Can you work these out from the model? Positions are in its coordinate system, mm. A direction names the side the tool comes from. Round coordinates to 2 decimals unless told otherwise and drop trailing zeros. Write each loop counter-clockwise with the first axis right and the second up, starting at its lowest first coordinate (ties: lowest second). Pieces come first, ordered by that corner, then holes. Notation, with made-up numbers: (-22.5, 67.5) - (27.5, 67.5) arc R19 ccw to (27.5, 88.5) - close; hole circle Ø4 at (44.5, 50.5). An arc over 180 degrees is marked (long way). One line per item, written item: value. Start each with the question number.
(1) If I drill on L1, parallel to X at y = 6.5, z = 93.5; L2, parallel to X at y = -48.1, z = 44, over which ranges is the centre line in solid material (lowest first)? Write a range as from..to.
(2) Thinking about a two-plate mould opening in Y: for faces 1 (the face through (-1, -47, 64)), 2 (the face through (-30, -49, 53)), 3 (the face through (-49.14, 49.1, 65.91)), which applies, +Y half, -Y half, draft (parallel to the pull), parting line (faces both ways), or undercut?
(3) I want a section at C-C on x = -3. List the corners of the cut face in (y, z) for me.
(4) I'm going to push flat-ended pins straight in: pin 1 Ø6 at (x, z) = (-34, 56) entering from +Y; pin 2 Ø5.5 at (y, z) = (35, 56) entering from -X. Where does each tip first touch, or does it pass through?
(5) I want a section at D-D on x = -32. List the corners of the cut face in (y, z) for me, plus the area to 3 significant figures.
(6) I want a section at A-A on x = -43. List the corners of the cut face in (y, z) for me.
(7) I want a section at B-B on z = 122. List the corners of the cut face in (x, y) for me, plus the area to 3 significant figures.
(8) On a 3-axis mill with a long thin cutter (end or side, diameter ignored), from which of +Z, -Z, +X, -X, +Y, -Y can I reach the whole of each face in a straight line? I mean faces 4 (the face through (49, -13, 30)), 5 (the face through (-48.521, 35.404, 59.074)), 6 (the face through (-11, 49, 118)). Say none if no direction works.
from build123d import *

# Parameters (mm, degrees)
SKETCH1_W                      = 100
SKETCH1_H                      = 100
SKETCH1_W_2                    = 94
SKETCH1_H_2                    = 94
EXTRUDE_THIN1_DEPTH            = 130
FILLET1_R                      = 0.5
FILLET2_R                      = 3
F_8_0_8_DIAMETER_HOLE2_D       = 8
F_8_0_8_DIAMETER_HOLE3_D       = 8
F_10_0_10_DIAMETER_HOLE1_D     = 10
F_10_0_10_DIAMETER_HOLE2_D     = 10
F_21_0_21_DIAMETER_HOLE1_D     = 42
F_21_0_21_DIAMETER_HOLE1_DEPTH = 3
F_6_0_6_DIAMETER_HOLE1_D       = 6
F_6_0_6_DIAMETER_HOLE1_DEPTH   = 3
SKETCH33_R                     = 4
CUT_EXTRUDE1_DEPTH             = 10
SKETCH34_R                     = 2
CUT_EXTRUDE2_DEPTH             = 10
SKETCH35_R                     = 2
CUT_EXTRUDE3_DEPTH             = 10
SKETCH36_R                     = 2
CUT_EXTRUDE4_DEPTH             = 10
SKETCH37_R                     = 2
CUT_EXTRUDE5_DEPTH             = 10
CUT_EXTRUDE6_REACH             = 173.464
SKETCH38_R                     = 3.1
CUT_EXTRUDE7_REACH             = 173.464
SKETCH39_R                     = 3.1


with BuildPart() as part:
    # Sketch1 → Extrude-Thin1 (new body)
    with BuildSketch(Plane.XY):
        Rectangle(SKETCH1_W, SKETCH1_H)
        Rectangle(SKETCH1_W_2, SKETCH1_H_2, mode=Mode.SUBTRACT)
    extrude(amount=EXTRUDE_THIN1_DEPTH)

    # Fillet1
    fillet1_edges = [part.edges().sort_by_distance(p)[0] for p in [
        (47, -47, 65),
        (47, 47, 65),
        (-47, 47, 65),
        (-47, -47, 65),
    ]]
    fillet(fillet1_edges, radius=FILLET1_R)

    # Fillet2
    fillet2_edges = [part.edges().sort_by_distance(p)[0] for p in [
        (50, -50, 65),
        (-50, -50, 65),
        (-50, 50, 65),
        (50, 50, 65),
    ]]
    fillet(fillet2_edges, radius=FILLET2_R)

    # Ø8.0 (8) Diameter Hole2 (through all)
    with Locations(Plane(origin=(0, 50, 0), x_dir=(1, 0, 0), z_dir=(0, 1, 0))):
        with Locations((28, -32), (28, -90)):
            Hole(F_8_0_8_DIAMETER_HOLE2_D / 2)

    # Ø8.0 (8) Diameter Hole3 (through all)
    with Locations(Plane(origin=(50, 0, 0), x_dir=(0, 0, -1), z_dir=(1, 0, 0))):
        with Locations((-14, 31), (-116, 31)):
            Hole(F_8_0_8_DIAMETER_HOLE3_D / 2)

    # Ø10.0 (10) Diameter Hole1 (through all)
    with Locations(Plane(origin=(0, 50, 0), x_dir=(1, 0, 0), z_dir=(0, 1, 0))):
        with Locations((-34, -56)):
            Hole(F_10_0_10_DIAMETER_HOLE1_D / 2)

    # Ø10.0 (10) Diameter Hole2 (through all)
    with Locations(Plane(origin=(50, 0, 0), x_dir=(0, 0, -1), z_dir=(1, 0, 0))):
        with Locations((-44, -31)):
            Hole(F_10_0_10_DIAMETER_HOLE2_D / 2)

    # Ø21.0 (21) Diameter Hole1
    with Locations(Plane(origin=(50, 0, 0), x_dir=(0, 0, -1), z_dir=(1, 0, 0))):
        with Locations((-70, 0)):
            Hole(F_21_0_21_DIAMETER_HOLE1_D / 2, depth=F_21_0_21_DIAMETER_HOLE1_DEPTH)

    # Ø6.0 (6) Diameter Hole1
    with Locations(Plane(origin=(50, 0, 0), x_dir=(0, 0, -1), z_dir=(1, 0, 0))):
        with Locations((-41.157258279, -16.652364697), (-53.347635303, 28.842741721), (-98.842741721, 16.652364697), (-86.652364697, -28.842741721)):
            Hole(F_6_0_6_DIAMETER_HOLE1_D / 2, depth=F_6_0_6_DIAMETER_HOLE1_DEPTH)

    # Sketch33 → Cut-Extrude1 (cut)
    with BuildSketch(Plane(origin=(0, 50, 0), x_dir=(1, 0, 0), z_dir=(0, 1, 0))):
        with Locations(Location((-3, -105, 0), (0, 0, 270))):
            Circle(SKETCH33_R)
    extrude(amount=-CUT_EXTRUDE1_DEPTH, mode=Mode.SUBTRACT)

    # Sketch34 → Cut-Extrude2 (cut)
    with BuildSketch(Plane(origin=(0, 50, 0), x_dir=(1, 0, 0), z_dir=(0, 1, 0))):
        with Locations(Location((-22, -14, 0), (0, 0, 270))):
            Circle(SKETCH34_R)
        with Locations(Location((-11, -14, 0), (0, 0, 270))):
            Circle(SKETCH34_R)
        with Locations(Location((-11, -116, 0), (0, 0, 90))):
            Circle(SKETCH34_R)
        with Locations(Location((-22, -116, 0), (0, 0, 90))):
            Circle(SKETCH34_R)
    extrude(amount=-CUT_EXTRUDE2_DEPTH, mode=Mode.SUBTRACT)

    # Sketch35 → Cut-Extrude3 (cut)
    with BuildSketch(Plane.ZY.offset(50)):
        with Locations(Location((56, 19, 0), (0, 0, 270))):
            Circle(SKETCH35_R)
        with Locations(Location((56, 8, 0), (0, 0, 270))):
            Circle(SKETCH35_R)
    extrude(amount=-CUT_EXTRUDE3_DEPTH, mode=Mode.SUBTRACT)

    # Sketch36 → Cut-Extrude4 (cut)
    with BuildSketch(Plane.XZ.offset(50)):
        with Locations(Location((16, 44, 0), (0, 0, 270))):
            Circle(SKETCH36_R)
        with Locations(Location((5, 44, 0), (0, 0, 270))):
            Circle(SKETCH36_R)
    extrude(amount=-CUT_EXTRUDE4_DEPTH, mode=Mode.SUBTRACT)

    # Sketch37 → Cut-Extrude5 (cut)
    with BuildSketch(Plane(origin=(50, 0, 0), x_dir=(0, 0, -1), z_dir=(1, 0, 0))):
        with Locations(Location((-32, -13, 0), (0, 0, 90))):
            Circle(SKETCH37_R)
        with Locations(Location((-32, -2, 0), (0, 0, 90))):
            Circle(SKETCH37_R)
        with Locations(Location((-94, -13, 0), (0, 0, 90))):
            Circle(SKETCH37_R)
        with Locations(Location((-94, -2, 0), (0, 0, 90))):
            Circle(SKETCH37_R)
    extrude(amount=-CUT_EXTRUDE5_DEPTH, mode=Mode.SUBTRACT)

    # Sketch38 → Cut-Extrude6 (cut, up to next)
    with BuildSketch(Plane.ZY.offset(50), mode=Mode.PRIVATE) as cut_extrude6_sk1:
        with Locations(Location((56, 35, 0), (0, 0, 270))):
            Circle(SKETCH38_R)
    cut_extrude6_tool1 = extrude(cut_extrude6_sk1.sketch, amount=-CUT_EXTRUDE6_REACH, mode=Mode.PRIVATE) & part.part
    # Sketch38 → Cut-Extrude6 (cut, up to next)
    with BuildSketch(Plane.ZY.offset(50), mode=Mode.PRIVATE) as cut_extrude6_sk2:
        with Locations(Location((56, -15, 0), (0, 0, 270))):
            Circle(SKETCH38_R)
    cut_extrude6_tool2 = extrude(cut_extrude6_sk2.sketch, amount=-CUT_EXTRUDE6_REACH, mode=Mode.PRIVATE) & part.part
    add(cut_extrude6_tool1.solids().sort_by_distance((-50, 35, 56))[0], mode=Mode.SUBTRACT)
    add(cut_extrude6_tool2.solids().sort_by_distance((-50, -15, 56))[0], mode=Mode.SUBTRACT)

    # Sketch39 → Cut-Extrude7 (cut, up to next)
    with BuildSketch(Plane.XZ.offset(50), mode=Mode.PRIVATE) as cut_extrude7_sk1:
        with Locations(Location((-20, 44, 0), (0, 0, 270))):
            Circle(SKETCH39_R)
    cut_extrude7_tool1 = extrude(cut_extrude7_sk1.sketch, amount=-CUT_EXTRUDE7_REACH, mode=Mode.PRIVATE) & part.part
    # Sketch39 → Cut-Extrude7 (cut, up to next)
    with BuildSketch(Plane.XZ.offset(50), mode=Mode.PRIVATE) as cut_extrude7_sk2:
        with Locations(Location((38, 44, 0), (0, 0, 270))):
            Circle(SKETCH39_R)
    cut_extrude7_tool2 = extrude(cut_extrude7_sk2.sketch, amount=-CUT_EXTRUDE7_REACH, mode=Mode.PRIVATE) & part.part
    add(cut_extrude7_tool1.solids().sort_by_distance((-20, -50, 44))[0], mode=Mode.SUBTRACT)
    add(cut_extrude7_tool2.solids().sort_by_distance((38, -50, 44))[0], mode=Mode.SUBTRACT)


solid = part.part
Established:
1. L1: -50..-47, 47..50
1. L2: -49.79..-23.1, -16.9..3, 7..14, 18..34.9, 41.1..49.79
2. face 1: undercut
2. face 2: draft
2. face 3: +Y half
3. outline: (-50, 0) - (-47, 0) - (-47, 130) - (-50, 130) - close; (47, 0) - (50, 0) - (50, 101) - (47, 101) - close; (47, 109) - (50, 109) - (50, 130) - (47, 130) - close
4. pin 1: through
4. pin 2: x = 47
5. outline: (-50, 0) - (-47, 0) - (-47, 51.42) - (-50, 51.42) - close; (-50, 60.58) - (-47, 60.58) - (-47, 130) - (-50, 130) - close; (47, 0) - (50, 0) - (50, 51.42) - (47, 51.42) - close; (47, 60.58) - (50, 60.58) - (50, 130) - (47, 130) - close
5. area: 725 mm2
6. outline: (-50, 0) - (-47, 0) - (-47, 130) - (-50, 130) - close; (47, 0) - (50, 0) - (50, 130) - (47, 130) - close
7. outline: (-50, -47) arc R3 ccw to (-47, -50) - (47, -50) arc R3 ccw to (50, -47) - (50, 47) arc R3 ccw to (47, 50) - (-47, 50) arc R3 ccw to (-50, 47) - close; hole (-47, -46.5) arc R0.5 ccw to (-46.5, -47) - (46.5, -47) arc R0.5 ccw to (47, -46.5) - (47, 46.5) arc R0.5 ccw to (46.5, 47) - (-46.5, 47) arc R0.5 ccw to (-47, 46.5) - close
7. area: 1,160 mm2
8. face 4: +X
8. face 5: -X
8. face 6: +Y
